Check sheet for the modelled part. Datum: model origin and axes. Units: mm. A direction names the side the tool comes from. Round coordinates to 2 decimals unless told otherwise and drop trailing zeros. Loops run counter-clockwise (first coordinate to the right, second up) from the corner with the lowest first, then second, coordinate; pieces in that order, holes last. Notation, with made-up numbers: (8, 3) - (60, 3) arc R34 ccw to (60, 38) - close; hole circle Ø7 at (-38, 71). An arc over 180 degrees is marked (long way). Put each result on its own line as item: value.
Autodesk Inventor part; units mm, degrees
ref_plane "YZ Plane" through (0, 0, 0) normal (1, 0, 0) x (0, 1, 0)
ref_plane "XZ Plane" through (0, 0, 0) normal (0, 1, 0) x (-1, 0, 0)
ref_plane "XY Plane" through (0, 0, 0) normal (0, 0, 1) x (1, 0, 0)
sketch "Sketch1" plane through (0, 0, 0) normal (0, 1, 0) x (-1, 0, 0)
  line L0 (0, 0) -> (0, -4.826)
  line L1 (0, -4.826) -> (0, 0)
  line L2 (0, 0) -> (0, 4.826)
  line L3 (0, 4.826) -> (9.1948, 4.826)
  line L4 (9.1948, -4.826) -> (0, -4.826)
  line L5 (9.1948, 4.826) -> (9.1948, 3.556)
  line L6 (9.1948, 3.556) -> (6.6548, 3.556)
  line L7 (9.1948, -4.826) -> (9.1948, -3.556)
  line L8 (9.1948, -3.556) -> (6.6548, -3.556)
  line L9 (9.1948, 4.826) -> (9.1948, 3.556)
  line L10 (9.1948, -3.556) -> (9.1948, -4.826)
  line L11 (9.1948, 0) -> (6.0198, 0)
  line L12 (5.6388, 0) -> (4.3688, 0)
  line L13 (4.3688, 0) -> (4.3688, -2.54)
  line L14 (4.3688, -2.54) -> (4.3688, 0)
  line L15 (4.3688, 0) -> (4.3688, 2.54)
  line L16 (4.3688, 2.54) -> (6.6548, 3.556)
  line L17 (4.3688, -2.54) -> (6.6548, -3.556)
  dimension "d0" = 4.826
  dimension "d1" = 4.826
  dimension "d2" = 9.1948
  dimension "d3" = 1.27
  dimension "d4" = 2.54
  dimension "d5" = 1.27
  dimension "d6" = 2.54
  dimension "d7" = 3.175
  dimension "d9" = 1.27
  dimension "d10" = 2.54
  dimension "d11" = 2.54
  dimension "d12" = 2.54
revolve "Revolution1" add sketch "Sketch1" angle 360 about axis through (0, 0, 0) along (0, 0, -1)
sketch "Sketch2" plane through (0, 0, -4.826) normal (0, 0, -1) x (-1, 0, 0)
  circle A0 centre (0, 0) radius 1.5875
  dimension "d14" = 3.175
extrude "Extrusion1" cut sketch "Sketch2" against normal through all
properties part number "updated_wheel"
Item 1: Section check C-C on z = 4. Enter the section's corners in (x, y) (1 decimal), then the cut area to 3 significant figures.
Filled sheet:
outline: circle Ø18.4 at (0, 0); hole circle Ø3.2 at (0, 0)
area: 258 mm²
Item 2: Tool access check on faces 4 (the flat face through (0, -2, -4.826)), 5 (the cylindrical face through (-4.167, -1.312, 0.036)). Record the directions out of +Z, -Z, +X, -X, +Y, -Y that give a thin tool (end or side, any length) a straight path to the whole face; none if there is none.
Filled sheet:
face 4: -Z, +X, -X, +Y, -Y
face 5: none
Item 3: Release check for a two-part mould opening along X. For faces 1 (the cylindrical face through (0.34, -1.55, -0.07)), 2 (the flat face through (-5, 5, 3.556)), 3 (the conical face through (-2.08, -4, -2.6)) record: +X half, -X half, draft (parallel to the pull), parting line (faces both ways), or undercut.
Filled sheet:
face 1: undercut
face 2: draft
face 3: parting line
Item 4: Section check D-D on y = 8. Enter the section's corners in (x, z), then the cut area to 3 significant figures.
Filled sheet:
outline: (-4.53, -4.83) - (4.53, -4.83) - (4.53, -3.56) - (-4.53, -3.56) - close; (-4.53, 3.56) - (4.53, 3.56) - (4.53, 4.83) - (-4.53, 4.83) - close
area: 23.0 mm²
Item 5: Thickness scan on line 1 (Y direction, x = 0, z = -1.5); line 2 (Z direction, x = -5.75, y = 3.75); line 3 (Y direction, x = 0, z = -3). Record the ranges inside material, lowest first. Write a range as from..to.
Filled sheet:
line 1: -4.37..-1.59, 1.59..4.37
line 2: -4.83..-3.56, 3.56..4.83
line 3: -5.4..-1.59, 1.59..5.4
Item 6: Section check A-A on y = 0. Enter the section's corners in (x, z), then the cut area to 3 significant figures.
Filled sheet:
outline: (-9.19, -4.83) - (-1.59, -4.83) - (-1.59, 4.83) - (-9.19, 4.83) - (-9.19, 3.56) - (-6.65, 3.56) - (-4.37, 2.54) - (-4.37, -2.54) - (-6.65, -3.56) - (-9.19, -3.56) - close; (1.59, -4.83) - (9.19, -4.83) - (9.19, -3.56) - (6.65, -3.56) - (4.37, -2.54) - (4.37, 2.54) - (6.65, 3.56) - (9.19, 3.56) - (9.19, 4.83) - (1.59, 4.83) - close
area: 82.9 mm²
Item 7: Go/stop test with flat-tipped pins: pin 1 (4 mm diameter, centred on y = -6.5, z = 3, fed in from -X); pin 2 (4 mm diameter, centred on x = 5.5, z = 0.5, fed in from +Y); pin 3 (2 mm diameter, centred on x = -2, z = -0.5, fed in from +Y). Record where each tip stops, or that it passes through.
Filled sheet:
pin 1: x = -7.97
pin 2: y = 2.61
pin 3: y = 4.25
